from build123d import *

# Parameters (mm, degrees)
SKETCH2_R             = 2.5
BOSS_EXTRUDE1_DEPTH   = 25.25
CHAMFER1_SIZE         = 0.1
CHAMFER1_SIZE2        = 0.173205081
CHAMFER1_PART_2_SIZE  = 0.1
CHAMFER1_PART_2_SIZE2 = 0.173205081
M3X0_5_TAPPED_HOLE1_D = 2.5


with BuildPart() as part:
    # Sketch2 → Boss-Extrude1 (new body)
    with BuildSketch(Plane(origin=(0, 0, 0), x_dir=(1, 0, 0), z_dir=(0, 1, 0))):
        Circle(SKETCH2_R)
    extrude(amount=BOSS_EXTRUDE1_DEPTH)

    # Chamfer1
    chamfer1_edges = [part.edges().sort_by_distance(p)[0] for p in [
        (-2.5, 0, 0),
    ]]
    chamfer1_side = [part.faces().sort_by_distance(p)[0] for p in [
        (0, 0, 0),
    ]]
    chamfer(chamfer1_edges, length=CHAMFER1_SIZE, length2=CHAMFER1_SIZE2, reference=chamfer1_side[0])

    # Chamfer1 part 2
    chamfer1_part_2_edges = [part.edges().sort_by_distance(p)[0] for p in [
        (-2.5, 25.25, 0),
    ]]
    chamfer1_part_2_side = [part.faces().sort_by_distance(p)[0] for p in [
        (-2.5, 12.625, 0),
    ]]
    chamfer(chamfer1_part_2_edges, length=CHAMFER1_PART_2_SIZE, length2=CHAMFER1_PART_2_SIZE2, reference=chamfer1_part_2_side[0])

    # M3x0.5 Tapped Hole1 (through all)
    with Locations(Plane(origin=(0, 25.25, 0), x_dir=(1, 0, 0), z_dir=(0, 1, 0))):
        with Locations((0, 0)):
            Hole(M3X0_5_TAPPED_HOLE1_D / 2)


solid = part.part
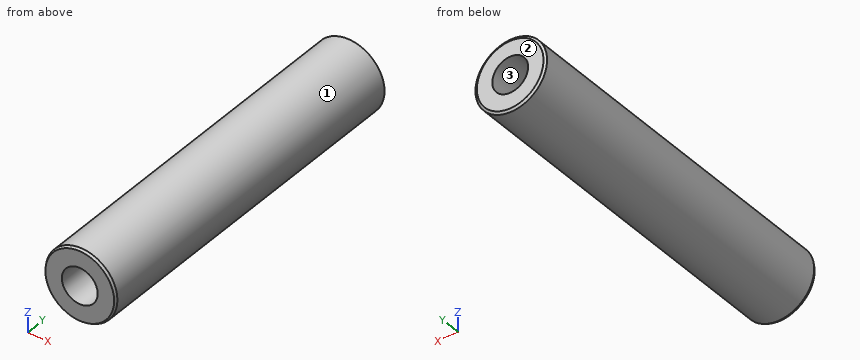
Read the model definition and answer for the solid it produces. Units are mm, in the model's axes. Face numbers are marked on the shaded views. Coordinates: 2 decimals unless noted, no trailing zeros. Loops run counter-clockwise (first coordinate to the right, second up) from the corner with the lowest first, then second, coordinate; pieces in that order, holes last. Notation, with made-up numbers: (33, 76) -> (67, 76) arc R33 cw to (67, 115) -> close; hole circle Ø2 at (51.25, -28). An arc over 180 degrees is marked (long way). Answer in a Markdown table with one row per item.
Item 1: A cutting plane is placed at A-A on x = 0. Determine the outline of the cut face in (y, z), plus the area to 3 significant figures.
Returned:
| item | result |
|---|---|
| outline | (0, -2.4) -> (0.17, -2.5) -> (25.15, -2.5) -> (25.25, -2.33) -> (25.25, -1.25) -> (0, -1.25) -> close; (0, 1.25) -> (25.25, 1.25) -> (25.25, 2.33) -> (25.15, 2.5) -> (0.17, 2.5) -> (0, 2.4) -> close |
| area | 63.1 mm^2 |
Item 2: For a pull along Z with two mould halves and no side action, classify the marked faces 1, 2 and 3 as released by +Z, released by -Z, zero draft, split by the parting line, or undercut.
Returned:
| item | result |
|---|---|
| face 1 | split by the parting line |
| face 2 | zero draft |
| face 3 | undercut |
Item 3: Straight lines are drawn through the part: line 1 along Z through (x, y) = (0, 23); line 2 along Z through (x, y) = (-0.85, 14.5); line 3 along X through (y, z) = (21.75, 1.1) (3 decimals). For each, find the intervals that lie inside material, in ascending order. Write a range as [from, to].
Returned:
| item | result |
|---|---|
| line 1 | z = [-2.5, -1.25], [1.25, 2.5] |
| line 2 | z = [-2.35, -0.92], [0.92, 2.35] |
| line 3 | x = [-2.245, -0.594], [0.594, 2.245] |
Item 4: A cutting plane is placed at C-C on y = 16.75. Determine the outline of the cut face in (x, z), plus the area to 3 significant figures.
Returned:
| item | result |
|---|---|
| outline | circle Ø5 at (0, 0); hole circle Ø2.5 at (0, 0) |
| area | 14.7 mm^2 |
Item 5: This flat-tipped pin is pushed along its axis until it touches: P1, Ø1.5, axis at y = 14, z = -1.5, coming from the -X side. Where does it stop, or does it pass through?
Returned:
| item | result |
|---|---|
| P1 | stops at x = -2.38 |
Item 6: A cutting plane is placed at B-B on z = 0. Determine the outline of the cut face in (x, y), plus the area to 3 significant figures.
Returned:
| item | result |
|---|---|
| outline | (-2.5, 0.17) -> (-2.4, 0) -> (-1.25, 0) -> (-1.25, 25.25) -> (-2.33, 25.25) -> (-2.5, 25.15) -> close; (1.25, 0) -> (2.4, 0) -> (2.5, 0.17) -> (2.5, 25.15) -> (2.33, 25.25) -> (1.25, 25.25) -> close |
| area | 63.1 mm^2 |
